```python
from build123d import *

# Parameters (mm, degrees)
PAD_DEPTH         = 9
SKETCH001_W       = 37.346859
SKETCH001_H       = 35.838272
POCKET_DEPTH      = 6
POCKET_DEPTH_BACK = 100
SKETCH002_R       = 2.5
POCKET001_DEPTH   = 38.001
SKETCH003_R       = 2.5
POCKET002_DEPTH   = 38.001


with BuildPart() as part:
    # Sketch → Pad (new body, symmetric)
    with BuildSketch(Plane.XY):
        Polygon((0, 0), (0, 38), (5, 38), (38, 5), (38, 0), align=None)
    extrude(amount=PAD_DEPTH, both=True)

    # Sketch001 → Pocket (cut, two sides)
    with BuildSketch(Plane.XY) as pocket_sk:
        with Locations((23.673429, 22.919136)):
            Rectangle(SKETCH001_W, SKETCH001_H)
    extrude(amount=-POCKET_DEPTH, mode=Mode.SUBTRACT)
    extrude(pocket_sk.sketch, amount=POCKET_DEPTH_BACK, mode=Mode.SUBTRACT)

    # Sketch002 (on Face2 of Pocket) → Pocket001 (cut, through all)
    with BuildSketch(Plane.XZ):
        with Locations((15, 0)):
            Circle(SKETCH002_R)
        with Locations((30, 0)):
            Circle(SKETCH002_R)
    extrude(amount=-POCKET001_DEPTH, mode=Mode.SUBTRACT)

    # Sketch003 (on Face1 of Pocket001) → Pocket002 (cut, through all)
    with BuildSketch(Plane(origin=(0, 0, 0), x_dir=(0, -1, 0), z_dir=(-1, 0, 0))):
        with Locations((-30, 0)):
            Circle(SKETCH003_R)
        with Locations((-15, 0)):
            Circle(SKETCH003_R)
    extrude(amount=-POCKET002_DEPTH, mode=Mode.SUBTRACT)


solid = part.part
```
Build history of the part. All positions in model axes, mm. A direction names the side the tool comes from. Coordinates: 2 decimals unless noted, no trailing zeros. Order: outer loops, then holes, each group sorted by start corner. A loop starts at its lowest first (then second) coordinate and runs counter-clockwise, first axis right, second up. Notation, with made-up numbers: (13, 38.5) -> (66, 38.5) arc R20 ccw to (66, 68.5) -> close; hole circle Ø7 at (70.25, 22). An arc over 180 degrees is marked (long way). Answer in a Markdown table with one row per item. Add a question column.
Q1. Band-saw the part on D-D, the plane x = 7. List the corners of the cut face in (y, z).
Q2. Mould opens along X. For faces 1 (the face through (27.5, 2.5, 0.1)), 2 (the face through (21, 22, -7)), 3 (the face through (2.5, 32.5, 0.1)) say: +X half, -X half, draft (parallel to the pull), parting line (faces both ways), or undercut.
Q3. Band-saw the part on A-A, the plane y = 30. List the corners of the cut face in (x, z), then the cut area to 3 significant figures.
Q4. Band-saw the part on B-B, the plane z = 0. List the corners of the cut face in (x, y).
Q5. Which spindle directions (+Z, -Z, +X, -X, +Y, -Y) get a long thin tool onto all of the face, cutting with end or side? Do faces 4 (the face through (19, 0, 0)), 5 (the face through (14, 18, -6)). Say none if no direction does.
Q6. Band-saw the part on C-C, the plane x = 15. List the corners of the cut face in (y, z).
Q7. Drop flat-ended pins along their axis: pin 1 (7.5 mm diameter, centred on y = 21.5, z = -1, fed in from +X); pin 2 (4 mm diameter, centred on x = 20, z = -2.5, fed in from +Y); pin 3 (16.5 mm diameter, centred on x = 23, y = 19.5, fed in from +Z). Give the stop position or say it passes through.
Q8. Wall check: line 1 along Y through (x, z) = (4.5, 0.75); line 2 along Z through (x, y) = (3.65, 30); line 3 along Y through (x, z) = (4.5, -1.5). Give the ranges that are in metal, low to high. Write a range as [from, to].
Answers follow:
| question | item | result |
|---|---|---|
| 1 | outline | (0, -9) -> (36, -9) -> (36, -6) -> (5, -6) -> (5, 9) -> (0, 9) -> close |
| 2 | face 1 | undercut |
| 2 | face 2 | +X half |
| 2 | face 3 | draft |
| 3 | outline | (0, -9) -> (13, -9) -> (13, -6) -> (5, -6) -> (5, -2.5) -> (0, -2.5) -> close; (0, 2.5) -> (5, 2.5) -> (5, 9) -> (0, 9) -> close |
| 3 | area | 89.0 mm^2 |
| 4 | outline | (0, 0) -> (12.5, 0) -> (12.5, 5) -> (5, 5) -> (5, 12.5) -> (0, 12.5) -> close; (0, 17.5) -> (5, 17.5) -> (5, 27.5) -> (0, 27.5) -> close; (0, 32.5) -> (5, 32.5) -> (5, 38) -> (0, 38) -> close; (17.5, 0) -> (27.5, 0) -> (27.5, 5) -> (17.5, 5) -> close; (32.5, 0) -> (38, 0) -> (38, 5) -> (32.5, 5) -> close |
| 5 | face 4 | +Z, -Z, +X, -X, -Y |
| 5 | face 5 | +Z, +X, +Y |
| 6 | outline | (0, -9) -> (28, -9) -> (28, -6) -> (5, -6) -> (5, -2.5) -> (0, -2.5) -> close; (0, 2.5) -> (5, 2.5) -> (5, 9) -> (0, 9) -> close |
| 7 | pin 1 | x = 5 |
| 7 | pin 2 | y = 5 |
| 7 | pin 3 | z = -6 |
| 8 | line 1 | [0, 12.62], [17.38, 27.62], [32.38, 38] |
| 8 | line 2 | [-9, -2.5], [2.5, 9] |
| 8 | line 3 | [0, 13], [17, 28], [32, 38] |
